Verification items for the finished model (mm, model axes). A direction names the side the tool comes from. Round coordinates to 2 decimals unless told otherwise and drop trailing zeros. Loops run counter-clockwise (first coordinate to the right, second up) from the corner with the lowest first, then second, coordinate; pieces in that order, holes last. Notation, with made-up numbers: (40.25, 43.5) - (79.25, 43.5) arc R13 cw to (79.25, 68.5) - close; hole circle Ø10 at (-37.75, 8). An arc over 180 degrees is marked (long way). Use a Markdown table: item, result. Add a question column.
Autodesk Inventor part; units mm, degrees
ref_plane "YZ Plane" through (0, 0, 0) normal (1, 0, 0) x (0, 1, 0)
ref_plane "XZ Plane" through (0, 0, 0) normal (0, 1, 0) x (-1, 0, 0)
ref_plane "XY Plane" through (0, 0, 0) normal (0, 0, 1) x (1, 0, 0)
sketch "Sketch1" plane through (0, 0, 0) normal (0, 1, 0) x (-1, 0, 0)
  circle A0 centre (0, 0) radius 3.5
  dimension "d0" = 7
extrude "Extrusion1" add sketch "Sketch1" along normal blind 4
sketch "Sketch2" plane through (0, 4, 0) normal (0, 1, 0) x (1, 0, 0)
  circle A0 centre (0, 0) radius 2
  dimension "d3" = 4
extrude "Extrusion2" add sketch "Sketch2" along normal blind 12
sketch "Sketch3" plane through (0, 0, 0) normal (0, -1, 0) x (1, 0, 0)
  line L0 (-1.7321, 0) -> (-0.866, 1.5)
  line L1 (-0.866, 1.5) -> (0.866, 1.5)
  line L2 (0.866, 1.5) -> (1.7321, 0)
  line L3 (1.7321, 0) -> (0.866, -1.5)
  line L4 (0.866, -1.5) -> (-0.866, -1.5)
  line L5 (-0.866, -1.5) -> (-1.7321, 0)
  point P0 (0, 0)
  point P1 (0, 0)
  dimension "d6" = 3
extrude "Extrusion3" cut sketch "Sketch3" against normal blind 2.7
thread "Thread1"
fillet "Fillet1" radius 0.3 1 edges at (-2, 16, 0)
fillet "Fillet2" radius 0.125 3 edges at (-2, 4, 0) (3.5, 4, 0) (3.5, 0, 0)
fillet "Fillet3" radius 0.05 13 edges at (-1.299, 0, -0.75) (-1.299, 0, 0.75) (0, 0, 1.5) (1.299, 0, 0.75) (1.299, 0, -0.75) (0.866, 1.35, -1.5) (0, 0, -1.5) (-1.299, 2.7, -0.75) (-1.299, 2.7, 0.75) (0, 2.7, 1.5) (1.299, 2.7, 0.75) (1.299, 2.7, -0.75) (0, 2.7, -1.5)
properties part number "MM-MMount_to_Motor-Bolt"
Q1. Section check C-C on y = 7. Record the cut outline in (x, z), plus the area to 3 significant figures.
Q2. Go/stop test with flat-tipped pins: pin 1 Ø2 at (y, z) = (13, 2) entering from +X; pin 2 Ø1 at (y, z) = (3.5, 2.5) entering from +X; pin 3 Ø4 at (x, y) = (2.5, 12) entering from -Z. Record where each tip stops, or that it passes through.
Q3. Release check for a two-part mould opening along X. For faces 3 (the face through (-2.2, 4, -0.7)), 4 (the face through (0, 10, -2)), 5 (the face through (1.31, 1.33, -0.73)) record: +X half, -X half, draft (parallel to the pull), parting line (faces both ways), or undercut.
Q4. Thickness scan on line 1 along Y through (x, z) = (-2.75, 0); line 2 along Y through (x, z) = (-1.5, 0.25); line 3 along Z through (x, y) = (0, 11). Record the ranges inside material, lowest first.
Q5. Section check B-B on x = 0. Record the cut outline in (y, z) (3 decimals).
Q6. Section check A-A on y = 1.5. Record the cut outline in (x, z) (3 decimals), plus the area to 3 significant figures.
Q7. Set-up check for faces 1 (the face through (-3.233, 1.974, 1.341)), 2 (the face through (0, 2.7, 0)): record each of +Z, -Z, +X, -X, +Y, -Y from which the full face is reachable in a straight line by a thin tool's end or side.
Determined:
| question | item | result |
|---|---|---|
| 1 | outline | circle Ø4 at (0, 0) |
| 1 | area | 12.6 mm² |
| 2 | pin 1 | stops at x = 1.73 |
| 2 | pin 2 | stops at x = 2.87 |
| 2 | pin 3 | stops at z = -1.94 |
| 3 | face 3 | draft |
| 3 | face 4 | parting line |
| 3 | face 5 | undercut |
| 4 | line 1 | y = 0 to 4 |
| 4 | line 2 | y = 2.7 to 16 |
| 4 | line 3 | z = -2 to 2 |
| 5 | outline | (0, -3.375) arc R0.125 ccw to (0.125, -3.5) - (3.875, -3.5) arc R0.125 ccw to (4, -3.375) - (4, -2.125) arc R0.125 cw to (4.125, -2) - (15.7, -2) arc R0.3 ccw to (16, -1.7) - (16, 1.7) arc R0.3 ccw to (15.7, 2) - (4.125, 2) arc R0.125 cw to (4, 2.125) - (4, 3.375) arc R0.125 ccw to (3.875, 3.5) - (0.125, 3.5) arc R0.125 ccw to (0, 3.375) - (0, 1.55) arc R0.05 ccw to (0.05, 1.5) - (2.65, 1.5) arc R0.05 cw to (2.7, 1.45) - (2.7, -1.45) arc R0.05 cw to (2.65, -1.5) - (0.05, -1.5) arc R0.05 ccw to (0, -1.55) - close |
| 6 | outline | circle Ø7 at (0, 0); hole (-1.732, 0) - (-0.866, -1.5) - (0.837, -1.5) arc R0.05 ccw to (0.88, -1.475) - (1.732, 0) - (0.866, 1.5) - (-0.866, 1.5) - close |
| 6 | area | 30.7 mm² |
| 7 | face 1 | +Y, -Y |
| 7 | face 2 | -Y |
